Can you work these out from the model? Positions are in its coordinate system, mm. A direction names the side the tool comes from. Give positions to 0.01 mm unless a question says otherwise; leave off trailing zeros. Loops run counter-clockwise (first coordinate to the right, second up) from the corner with the lowest first, then second, coordinate; pieces in that order, holes last. Notation, with made-up numbers: (-39, 4.5) -> (17, 4.5) arc R14 ccw to (17, 25.5) -> close; hole circle Ø1 at (87.5, -8.75). An arc over 180 degrees is marked (long way). One line per question, with ' | ' between items.
Autodesk Inventor part; units mm, degrees
ref_plane "Work Plane1" through (0, -17.5, 0) normal (1, 0, 0) x (0, 0, 1)
ref_plane "YZ Plane" through (0, 0, 0) normal (1, 0, 0) x (0, 1, 0)
ref_plane "XZ Plane" through (0, 0, 0) normal (0, 1, 0) x (-1, 0, 0)
sketch "Эскиз1" plane through (0, 0, 0) normal (0, 0, 1) x (1, 0, 0)
  line L0 (-6, 0) -> (6, 0) construction
  arc A0 (0.625, -33.9882) -> (-0.625, -33.9882) centre (0, -17.5) ccw
  line L1 (0, 20.1894) -> (0, -80.5364)
  line L2 (-48.09, 0) -> (48.09, 0)
  line L3 (-0.625, -33.9882) -> (-0.625, -39.5882)
  line L4 (-0.625, -6.5402) -> (-0.625, -13.29) construction
  line L5 (-2.7947, 3.9) -> (3.6722, 3.9) construction
  arc A1 (6.5262, -35.8793) -> (-6.5262, -35.8793) centre (0, -16.525) ccw
  arc A2 (-2.8189, -39.4165) -> (-0.625, -39.5882) centre (0, -17.5) ccw
  arc A3 (-4.9125, -37.5926) -> (-2.8189, -39.4165) centre (-2.5, -36.9369) ccw
  arc A4 (-4.9125, -37.5926) -> (-6.5262, -35.8793) centre (-7.325, -38.2483) ccw
  line L6 (0.625, -33.9882) -> (0.625, -39.5882)
  line L7 (0.625, -6.5402) -> (0.625, -13.29) construction
  arc A5 (0.625, -39.5882) -> (2.8189, -39.4165) centre (0, -17.5) ccw
  arc A6 (2.8189, -39.4165) -> (4.9125, -37.5926) centre (2.5, -36.9369) ccw
  arc A7 (6.5262, -35.8793) -> (4.9125, -37.5926) centre (7.325, -38.2483) ccw
  circle A8 centre (-2.5, -36.9369) radius 1.25
  circle A9 centre (2.5, -36.9369) radius 1.25
  dimension "d0" = 33
  dimension "d1" = 5.6
  dimension "d6" = 0.625
  dimension "d7" = 3.9
  dimension "d8" = 0.975
  dimension "d9" = 2.5
  dimension "d10" = 2.5
  dimension "d11" = 1.875
  dimension "d12" = 2.5
  dimension "d13" = 2.5
  dimension "d14" = 17.5
extrude "Базовый элемент" add sketch "Эскиз1" along normal blind 1.7
ref_plane "Work Plane1" through (0, -17.5, 0) normal (1, 0, 0) x (0, 0, 1)
equation "\"d0\" = ND"
equation "\"d1\" = SRB2"
equation "\"d6\" = 0.25 * SD5"
equation "\"d7\" = SRB1"
equation "\"d8\" = 0.25 * SRB1"
equation "\"d9\" = SD5"
equation "\"d10\" = SD5"
equation "\"d11\" = 0.75 * SD5"
equation "\"d12\" = SD5"
equation "\"d13\" = SD5"
equation "\"d14\" = 0.5 * WD"
equation "\"d2\" = SD"
equation "\"WD\" = WDMIN"
equation "\"SD\" = 1.7"
equation "\"SRB1\" = 3.9"
equation "\"ND\" = 33"
equation "\"SRB2\" = 5.6"
equation "\"SD5\" = 2.5"
equation "\"WDMIN\" = 35"
equation "\"SD3\" = 32.2"
equation "\"WDMAX\" = 36"
equation "\"SNB\" = 1.9"
equation "\"BUBRMI\" = 3"
properties part number "Кольцо A35 ГОСТ 13942-86" material "Сталь, мягкая"
Q1. If we mould it in two halves opening along Y, with no side actions, what happens to faces 3 (the face through (4.158, -38.808, 0.838)), 4 (the face through (2.337, -38.176, 0.838)), 5 (the face through (0.625, -37, 1))? For each: pulls with the +Y half, pulls with the -Y half, needs draft (parallel to the pull), parting line crosses it, or undercut.
Entries:
face 3: pulls with the -Y half | face 4: undercut | face 5: needs draft
Q2. If we section it at D-D (x = 0): Write out the boundary of the cut face in (y, z).
Entries:
outline: (-1, 0) -> (3.9, 0) -> (3.9, 1.7) -> (-1, 1.7) -> close
Q3. For pin 1 Ø5 at (x, y) = (-9, -26.5) entering from -Z; pin 2 Ø1 at (x, z) = (-8.5, 1) entering from +Y; pin 3 Ø0.5 at (y, z) = (-37, 1) entering from +X, each with a flat end and sliding along its axis, tell me the tip position at first contact or that it passes through.
Entries:
pin 1: through | pin 2: y = 2.27 | pin 3: x = 5.32
Q4. On a 3-axis mill with a long thin cutter (end or side, diameter ignored), from which of +Z, -Z, +X, -X, +Y, -Y can I reach the whole of each face in a straight line? I mean faces 1 (the face through (-0.625, -37, 1)), 2 (the face through (-5.52, -36.52, 0.84)). Say none if no direction works.
Entries:
face 1: +Z, -Z, -Y | face 2: +Z, -Z, -X, -Y
Q5. If we section it at C-C (z = 0.7): State how many separate pieces and enclosed holes the cut face has, plus the area to 3 significant figures.
Entries:
separate pieces: 1 | enclosed holes: 2 | area: 464 mm²
Q6. If I drill on probe 1 along Y at (x, z) = (3, 1.2); probe 2 along Y at (x, z) = (-2.5, 0.85); probe 3 along Y at (x, z) = (0, 0.6), over which ranges is the centre line in solid material (lowest first)? Write a range as from..to.
Entries:
probe 1: -39.39..-38.08, -35.79..-33.73, -1.27..3.68 | probe 2: -39.46..-38.19, -35.69..-33.81, -1.19..3.75 | probe 3: -1..3.9
Q7. If we section it at A-A (y = -29.5): Write out the boundary of the cut face in (x, z), plus the area to 3 significant figures.
Entries:
outline: (-15.77, 0) -> (-11.32, 0) -> (-11.32, 1.7) -> (-15.77, 1.7) -> close; (11.32, 0) -> (15.77, 0) -> (15.77, 1.7) -> (11.32, 1.7) -> close | area: 15.1 mm²
Q8. If we section it at B-B (x = -5.5): Write out the boundary of the cut face in (y, z), plus the area to 3 significant figures.
Entries:
outline: (-36.54, 0) -> (-33.06, 0) -> (-33.06, 1.7) -> (-36.54, 1.7) -> close; (-1.94, 0) -> (3.15, 0) -> (3.15, 1.7) -> (-1.94, 1.7) -> close | area: 14.6 mm²
